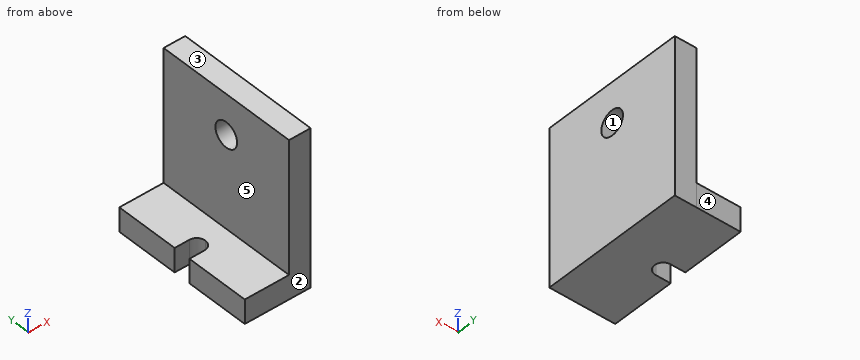
from build123d import *

# Parameters (mm, degrees)
F1_DEPTH = 66.04
F0_W     = 18.697526
F0_H     = 30.504273
F0_H_2   = 30.559674
F2_DEPTH = 10.16
F3_R     = 5.279602
F4_DEPTH = 25.4
F6_DEPTH = 25.4


with BuildPart() as f1:
    # F0 (on Top) → F1 (new body)
    with BuildSketch(Plane.XY):
        Polygon((0, 30.504273), (0, 0), (0, -30.559674), (9.12961, -30.559674), (9.12961, 30.504273), align=None)
    extrude(amount=F1_DEPTH)

    # F0 (on Top) → F2 (join)
    with BuildSketch(Plane.XY):
        with Locations((-9.348763, 15.252136)):
            Rectangle(F0_W, F0_H)
        with Locations((-9.348763, -15.279837)):
            Rectangle(F0_W, F0_H_2)
    extrude(amount=F2_DEPTH)

    # F3 (on face) → F4 (cut)
    with BuildSketch(Plane.YZ.offset(9.12961)):
        with Locations((0, 49.131077)):
            Circle(F3_R)
    extrude(amount=-F4_DEPTH, mode=Mode.SUBTRACT)

    # F5 (on face) → F6 (cut)
    with BuildSketch(Plane.XY.offset(10.16)):
        with BuildLine():
            ThreePointArc((-12.458752, -3.593451), (-9.917798, -2.540954), (-8.8653, 0))
            ThreePointArc((-8.8653, 0), (-9.917798, 2.540954), (-12.458752, 3.593451))
            Line((-12.458752, 3.593451), (-12.458752, 0))
            Line((-12.458752, 0), (-12.458752, -3.593451))
        make_face()
        with BuildLine():
            Line((-12.458752, 0), (-12.458752, 3.593451))
            ThreePointArc((-12.458752, 3.593451), (-16.052203, 0), (-12.458752, -3.593451))
            Line((-12.458752, -3.593451), (-12.458752, 0))
        make_face()
        with BuildLine():
            ThreePointArc((-12.458752, -3.593451), (-16.052203, 0), (-12.458752, 3.593451))
            Line((-12.458752, 3.593451), (-18.697526, 3.593451))
            Line((-18.697526, 3.593451), (-18.697526, -3.593451))
            Line((-18.697526, -3.593451), (-12.458752, -3.593451))
        make_face()
    extrude(amount=-F6_DEPTH, mode=Mode.SUBTRACT)


solid = f1.part
Design review of the part built by this model. Coordinates are the model's own, in mm. Face numbers are marked on the shaded views. A direction names the side the tool comes from. Coordinates: 2 decimals unless noted, no trailing zeros. Write each loop counter-clockwise with the first axis right and the second up, starting at its lowest first coordinate (ties: lowest second). Pieces come first, ordered by that corner, then holes. Notation, with made-up numbers: (25, 27) - (37, 27) arc R23 ccw to (37, 61) - close; hole circle Ø6 at (36, 22.25). An arc over 180 degrees is marked (long way). Use one line per item in the form item = value.
Q1. Insertion check: pin 1 Ø5 at (y, z) = (-6, 53) entering from -X; pin 2 Ø15 at (x, y) = (-9.5, 7) entering from +Z; pin 3 Ø9.5 at (y, z) = (0, 49.13) entering from -X. Each pin has a flat end and moves straight along its axis. Give the tip position at first contact, or say it passes through.
Taken from the geometry:
pin_1 = 0
pin_2 = 10.16
pin_3 = through
Q2. Consider section A-A (z = 50). Write out the cut boundary in (x, y).
Taken from the geometry:
outline = (0, -30.56) - (9.13, -30.56) - (9.13, -5.21) - (0, -5.21) - close; (0, 5.21) - (9.13, 5.21) - (9.13, 30.5) - (0, 30.5) - close
Q3. Consider section D-D (x = -6.5). Write out the cut boundary in (y, z), plus the area to 3 significant figures.
Taken from the geometry:
outline = (-30.56, 0) - (30.5, 0) - (30.5, 10.16) - (-30.56, 10.16) - close
area = 620 mm^2
Q4. Consider section B-B (y = -20.5). Write out the cut boundary in (x, z), plus the area to 3 significant figures.
Taken from the geometry:
outline = (-18.7, 0) - (9.13, 0) - (9.13, 66.04) - (0, 66.04) - (0, 10.16) - (-18.7, 10.16) - close
area = 793 mm^2
Q5. For probe 1 along Z at (x, y) = (6.5, 0); probe 2 along Z at (x, y) = (-15.5, 16.5); probe 3 along X at (y, z) = (8, 58), list the stretches that pass through material, from the lowest coordinate up.
Taken from the geometry:
probe_1 = 0 to 43.85, 54.41 to 66.04
probe_2 = 0 to 10.16
probe_3 = 0 to 9.13
Q6. Machinability: for the marked faces 4 and 5, which of the approach directions +Z, -Z, +X, -X, +Y, -Y give a long, thin tool a straight path to every point of the face, cutting with its end or side? Answer none if there is none.
Taken from the geometry:
face_4 = +Z, -Z, +X, -X, +Y
face_5 = +Z, -X, +Y, -Y
Q7. Consider section C-C (x = 3.5). Write out the cut boundary in (y, z), plus the area to 3 significant figures.
Taken from the geometry:
outline = (-30.56, 0) - (30.5, 0) - (30.5, 66.04) - (-30.56, 66.04) - close; hole circle Ø10.56 at (0, 49.13)
area = 3,950 mm^2
Q8. The part is to be moulded in two halves that separate along Z. For the marked faces 1, 2 and 3, say which applies: +Z half, -Z half, draft (parallel to the pull), parting line (faces both ways), or undercut.
Taken from the geometry:
face_1 = undercut
face_2 = draft
face_3 = +Z half
